Autodesk Inventor part; units mm, degrees
ref_plane "YZ Plane" through (0, 0, 0) normal (1, 0, 0) x (0, 1, 0)
ref_plane "XZ Plane" through (0, 0, 0) normal (0, 1, 0) x (-1, 0, 0)
ref_plane "XY Plane" through (0, 0, 0) normal (0, 0, 1) x (1, 0, 0)
sketch "Sketch1" plane through (0, 0, 0) normal (0, 1, 0) x (-1, 0, 0)
  line L0 (200, 400) -> (-200, 400)
  line L1 (-200, 400) -> (-200, -400)
  line L2 (-200, -400) -> (200, -400)
  line L3 (200, -400) -> (200, 400)
  line L4 (65.5, -226.6667) -> (-65.5, -226.6667)
  line L5 (-65.5, -226.6667) -> (-65.5, -306.6667)
  line L6 (-65.5, -306.6667) -> (65.5, -306.6667)
  line L7 (65.5, -306.6667) -> (65.5, -226.6667)
  point P0 (0, 0)
  dimension "d0" = 800
  dimension "d1" = 400
  dimension "d3" = 200
  dimension "d4" = 400
  dimension "d5" = 80
  dimension "d6" = 131
  dimension "d7" = 134.5
  dimension "d8" = 93.3333
sketch "Sketch2" plane through (0, 0, 0) normal (0, 1, 0) x (-1, 0, 0)
  point P0 (0, 0)
sketch "Sketch3" plane through (0, 0, 0) normal (1, 0, 0) x (0, 1, 0)
  point P0 (0, 0)
sketch "Sketch4" plane through (0, 0, 0) normal (0, 1, 0) x (-1, 0, 0)
  point P0 (0, 0)
  point P1 (0, 0)
sketch "Sketch5" plane through (0, 0, 0) normal (0, 1, 0) x (-1, 0, 0)
  point P0 (0, 0)
extrude "Extrusion1" add sketch "Sketch1" along normal mid plane 4
equation "\"d7\" = 0.5 * d1 - 0.5 * d6"
equation "\"d8\" = 0.166667 * d0 - 0.5 * d5"
properties part number "front"
For this review, take the finished solid that the model builds, in its own axes (mm). Coordinates: 2 decimals unless noted, no trailing zeros. Write each loop counter-clockwise with the first axis right and the second up, starting at its lowest first coordinate (ties: lowest second). Pieces come first, ordered by that corner, then holes.
(1) Wall thickness on probe 1 along X at (y, z) = (1.25, -252); probe 2 along Z at (x, y) = (-29, 0.7): over which ranges is each line inside the solid? List them lowest first.
(2) Add section A-A on x = 6. Give the boundary of the cut face in (y, z), then the cut area to 3 significant figures.
(3) Add section B-B on y = -1.1. Give the boundary of the cut face in (x, z), then the cut area to 3 significant figures.
Answer sheet:
1. probe 1: x = -200 to -65.5, 65.5 to 200
1. probe 2: z = -400 to -306.67, -226.67 to 400
2. outline: (-2, -400) - (2, -400) - (2, -306.67) - (-2, -306.67) - close; (-2, -226.67) - (2, -226.67) - (2, 400) - (-2, 400) - close
2. area: 2,880 mm2
3. outline: (-200, -400) - (200, -400) - (200, 400) - (-200, 400) - close; hole (-65.5, -306.67) - (65.5, -306.67) - (65.5, -226.67) - (-65.5, -226.67) - close
3. area: 310,000 mm2
